```python
from build123d import *

# Parameters (mm, degrees)
F_1_4_CLEARANCE_HOLE1_D = 6.5278
SKETCH4_W               = 12.7
SKETCH4_H               = 12.7
CUT_EXTRUDE1_DEPTH      = 0.127


with BuildPart() as part:
    # Sketch1 → Revolve1 (revolve)
    with BuildSketch(Plane(origin=(0, 0, 0), x_dir=(0, 0, -1), z_dir=(1, 0, 0))):
        Polygon((-6.35, 0), (-6.35, 4.2545), (-3.429, 6.35), (0, 6.35), (0, 0), align=None)
    revolve(axis=Axis((0, 0, 0), (0, 0, 1)))

    # 1/4 Clearance Hole1 (through all)
    with Locations(Plane.XY.offset(6.35)):
        with Locations((0, 0)):
            Hole(F_1_4_CLEARANCE_HOLE1_D / 2)

    # Sketch4 → Cut-Extrude1 (cut)
    with BuildSketch(Plane(origin=(0, 0, 0), x_dir=(-1, 0, 0), z_dir=(0, 0, -1))):
        Rectangle(SKETCH4_W, SKETCH4_H)
    extrude(amount=-CUT_EXTRUDE1_DEPTH, mode=Mode.SUBTRACT)


solid = part.part
```
The model under review builds one solid part; all positions refer to its coordinate system, in mm. Coordinates: 2 decimals unless noted, no trailing zeros. Order: outer loops, then holes, each group sorted by start corner. A loop starts at its lowest first (then second) coordinate and runs counter-clockwise, first axis right, second up. Notation, with made-up numbers: (-34.75, 37.25) -> (3.25, 37.25) arc R10 ccw to (3.25, 48.25) -> close; hole circle Ø1 at (40.5, 3). An arc over 180 degrees is marked (long way). Answer in a Markdown table with one row per item. Add a question column.
Item 1: We need section C-C on z = 0.5. Write out the cut boundary in (x, y), plus the area to 3 significant figures.
Item 2: We need section A-A on x = 0. Write out the cut boundary in (y, z).
Item 3: To check wall thickness, follow probe 1 along Y at (x, z) = (0, 2); probe 2 along Y at (x, z) = (2.25, 5); probe 3 along X at (y, z) = (0.75, 3.5). State the ranges of each line that lie inside material, in increasing order.
Item 4: Mouldability with a two-part tool opening along X and no side actions: class faces 1 (the conical face through (4.28, -0.95, 6.17)), 2 (the cylindrical face through (0.708, -3.186, 3.195)), 3 (the flat face through (3, -2, 6.35)) as +X half, -X half, draft (parallel to the pull), parting line (faces both ways), or undercut.
Item 5: We need section D-D on z = 5.5. Write out the cut boundary in (x, y).
Item 6: Clearance check with flat-ended pins moving along their axes: pin 1 (1 mm diameter, centred on x = -2.5, y = -4.5, fed in from +Z); pin 2 (1 mm diameter, centred on y = 2.5, z = 1, fed in from +X); pin 3 (6 mm diameter, centred on x = 0, y = 0, fed in from -Z); pin 4 (1 mm diameter, centred on y = 5, z = 1, fed in from -X). State where each tip first meets the part, or that it passes through.
Final values:
| question | item | result |
|---|---|---|
| 1 | outline | circle Ø12.7 at (0, 0); hole circle Ø6.53 at (0, 0) |
| 1 | area | 93.2 mm2 |
| 2 | outline | (-6.35, 0.13) -> (-3.26, 0.13) -> (-3.26, 6.35) -> (-4.25, 6.35) -> (-6.35, 3.43) -> close; (3.26, 0.13) -> (6.35, 0.13) -> (6.35, 3.43) -> (4.25, 6.35) -> (3.26, 6.35) -> close |
| 3 | probe 1 | y = -6.35 to -3.26, 3.26 to 6.35 |
| 3 | probe 2 | y = -4.71 to -2.36, 2.36 to 4.71 |
| 3 | probe 3 | x = -6.25 to -3.18, 3.18 to 6.25 |
| 4 | face 1 | parting line |
| 4 | face 2 | undercut |
| 4 | face 3 | draft |
| 5 | outline | circle Ø9.73 at (0, 0); hole circle Ø6.53 at (0, 0) |
| 6 | pin 1 | stops at z = 5.8 |
| 6 | pin 2 | stops at x = 6.03 |
| 6 | pin 3 | passes through |
| 6 | pin 4 | stops at x = -4.48 |
